The listing builds one solid part. Answer for the finished solid, in the listing's coordinates (mm). A direction names the side the tool comes from. Give positions to 0.01 mm unless a question says otherwise; leave off trailing zeros. Loops run counter-clockwise (first coordinate to the right, second up) from the corner with the lowest first, then second, coordinate; pieces in that order, holes last. Notation, with made-up numbers: M 47,39 L 84,39 A12 ccw 84,56 Z; hole C 83.5,62.5 d1. An arc over 180 degrees is marked long. One line per item, written item: value. Start each with the question number.
Q1. For faces 1 (the flat face through (77, 150, 3)), 2 (the flat face through (79, 170, 2)), determine the directions among +Z, -Z, +X, -X, +Y, -Y from which every point of the face is accessible in a straight line to the end or side of a thin tool.
Q2. A flat-ended cylindrical pin translates along its axis: pin 1 (4 mm diameter, centred on x = 160, y = 100, fed in from +Z). Find the tip coordinate at first contact, or state that the pin passes through.
Q3. A cutting plane is placed at B-B, the plane y = 22. Determine the outline of the cut face in (x, z).
Q4. Consider L1, parallel to X at y = 87.5, z = 2.6; L2, parallel to X at y = 132, z = 4.2; L3, parallel to Y at x = 40, z = 2.95. Determine where each line is inside the solid, lowest interval first.
Q5. The mould has two halves that part along X. Classify faces 3 (the flat face through (-15, 71, 2)), 4 (the flat face through (120, 69, 5)), 5 (the flat face through (45, 69, 3)): +X half, -X half, draft (parallel to the pull), parting line (faces both ways), or undercut.
Q6. A cutting plane is placed at C-C, the plane z = 2.95. State how many separate pieces and enclosed holes the cut face has, and give its area (3 significant figures).
Q7. A cutting plane is placed at A-A, the plane x = 56.5. Determine the outline of the cut face in (y, z), and give its area (3 significant figures).
from build123d import *

# Parameters (mm, degrees)
SKETCH_1_W          = 170
SKETCH_1_H          = 140
EXTRUDE_1_DEPTH     = 5
CUT_EXTRUDE_1_DEPTH = 5
SKETCH_4_R          = 1.6
CUT_EXTRUDE_2_DEPTH = 5
SKETCH_9_W          = 170
SKETCH_9_H          = 5
EXTRUDE_2_DEPTH     = 30
SKETCH_10_W         = 170
SKETCH_10_H         = 5
EXTRUDE_3_DEPTH     = 30
SKETCH_8_W          = 65
SKETCH_8_H          = 160
CUT_EXTRUDE_5_DEPTH = 30
SKETCH_6_R          = 1.75
CUT_EXTRUDE_6_DEPTH = 30
SKETCH_13_W         = 5
SKETCH_13_H         = 200
EXTRUDE_4_DEPTH     = 15
SKETCH_14_R         = 1.75
CUT_EXTRUDE_7_DEPTH = 15


with BuildPart() as part:
    # 草图1 → 凸台-拉伸1 (new body)
    with BuildSketch(Plane.XY):
        with Locations((85, 70)):
            Rectangle(SKETCH_1_W, SKETCH_1_H)
    extrude(amount=EXTRUDE_1_DEPTH)

    # 草图3 → 切除-拉伸1 (cut)
    with BuildSketch(Plane.XY.offset(5)):
        with BuildLine():
            ThreePointArc((10, 128.4), (11.13137085, 128.86862915), (11.6, 130))
            Line((11.6, 130), (10, 130))
            Line((10, 130), (10, 128.4))
        make_face()
        with BuildLine():
            Line((10, 130), (11.6, 130))
            ThreePointArc((11.6, 130), (8.86862915, 131.13137085), (10, 128.4))
            Line((10, 128.4), (10, 130))
        make_face()
        with BuildLine():
            ThreePointArc((10, 128.4), (11.13137085, 128.86862915), (11.6, 130))
            Line((11.6, 130), (10, 130))
            Line((10, 130), (10, 128.4))
        make_face()
        with BuildLine():
            Line((10, 130), (11.6, 130))
            ThreePointArc((11.6, 130), (8.86862915, 131.13137085), (10, 128.4))
            Line((10, 128.4), (10, 130))
        make_face()
        with BuildLine():
            ThreePointArc((11.6, 10), (11.13137085, 11.13137085), (10, 11.6))
            Line((10, 11.6), (10, 10))
            Line((10, 10), (11.6, 10))
        make_face()
        with BuildLine():
            Line((10, 10), (10, 11.6))
            ThreePointArc((10, 11.6), (8.86862915, 8.86862915), (11.6, 10))
            Line((11.6, 10), (10, 10))
        make_face()
        with BuildLine():
            ThreePointArc((11.6, 10), (11.13137085, 11.13137085), (10, 11.6))
            Line((10, 11.6), (10, 10))
            Line((10, 10), (11.6, 10))
        make_face()
        with BuildLine():
            Line((10, 10), (10, 11.6))
            ThreePointArc((10, 11.6), (8.86862915, 8.86862915), (11.6, 10))
            Line((11.6, 10), (10, 10))
        make_face()
        with BuildLine():
            ThreePointArc((161.6, 10), (161.13137085, 11.13137085), (160, 11.6))
            Line((160, 11.6), (160, 10))
            Line((160, 10), (158.4, 10))
            ThreePointArc((158.4, 10), (160, 8.4), (161.6, 10))
        make_face()
        with BuildLine():
            Line((160, 10), (160, 11.6))
            ThreePointArc((160, 11.6), (158.86862915, 11.13137085), (158.4, 10))
            Line((158.4, 10), (160, 10))
        make_face()
        with BuildLine():
            ThreePointArc((161.6, 10), (161.13137085, 11.13137085), (160, 11.6))
            Line((160, 11.6), (160, 10))
            Line((160, 10), (158.4, 10))
            ThreePointArc((158.4, 10), (160, 8.4), (161.6, 10))
        make_face()
        with BuildLine():
            Line((160, 10), (160, 11.6))
            ThreePointArc((160, 11.6), (158.86862915, 11.13137085), (158.4, 10))
            Line((158.4, 10), (160, 10))
        make_face()
        with BuildLine():
            ThreePointArc((161.6, 130), (160, 131.6), (158.4, 130))
            Line((158.4, 130), (160, 130))
            Line((160, 130), (160, 128.4))
            ThreePointArc((160, 128.4), (161.13137085, 128.86862915), (161.6, 130))
        make_face()
        with BuildLine():
            Line((160, 130), (158.4, 130))
            ThreePointArc((158.4, 130), (158.86862915, 128.86862915), (160, 128.4))
            Line((160, 128.4), (160, 130))
        make_face()
        with BuildLine():
            ThreePointArc((161.6, 130), (160, 131.6), (158.4, 130))
            Line((158.4, 130), (160, 130))
            Line((160, 130), (160, 128.4))
            ThreePointArc((160, 128.4), (161.13137085, 128.86862915), (161.6, 130))
        make_face()
        with BuildLine():
            Line((160, 130), (158.4, 130))
            ThreePointArc((158.4, 130), (158.86862915, 128.86862915), (160, 128.4))
            Line((160, 128.4), (160, 130))
        make_face()
    extrude(amount=-CUT_EXTRUDE_1_DEPTH, mode=Mode.SUBTRACT)

    # 草图4 → 切除-拉伸2 (cut)
    with BuildSketch(Plane.XY.offset(5)):
        with Locations((10, 130)):
            Circle(SKETCH_4_R)
        with Locations((40, 130)):
            Circle(SKETCH_4_R)
        with Locations((70, 130)):
            Circle(SKETCH_4_R)
        with Locations((100, 130)):
            Circle(SKETCH_4_R)
        with Locations((130, 130)):
            Circle(SKETCH_4_R)
        with Locations((10, 10)):
            Circle(SKETCH_4_R)
        with Locations((40, 10)):
            Circle(SKETCH_4_R)
        with Locations((70, 10)):
            Circle(SKETCH_4_R)
        with Locations((100, 10)):
            Circle(SKETCH_4_R)
        with Locations((130, 10)):
            Circle(SKETCH_4_R)
        with Locations((160, 130)):
            Circle(SKETCH_4_R)
        with Locations((10, 100)):
            Circle(SKETCH_4_R)
        with Locations((160, 100)):
            Circle(SKETCH_4_R)
        with Locations((10, 70)):
            Circle(SKETCH_4_R)
        with Locations((160, 70)):
            Circle(SKETCH_4_R)
        with Locations((10, 40)):
            Circle(SKETCH_4_R)
        with Locations((160, 40)):
            Circle(SKETCH_4_R)
    extrude(amount=-CUT_EXTRUDE_2_DEPTH, mode=Mode.SUBTRACT)

    # 草图9 → 凸台-拉伸2 (add)
    with BuildSketch(Plane.XZ):
        with Locations((85, 2.5)):
            Rectangle(SKETCH_9_W, SKETCH_9_H)
    extrude(amount=EXTRUDE_2_DEPTH)

    # 草图10 → 凸台-拉伸3 (add)
    with BuildSketch(Plane(origin=(0, 140, 0), x_dir=(1, 0, 0), z_dir=(0, 1, 0))):
        with Locations((85, -2.5)):
            Rectangle(SKETCH_10_W, SKETCH_10_H)
    extrude(amount=EXTRUDE_3_DEPTH)

    # 草图8 → 切除-拉伸5 (cut)
    with BuildSketch(Plane.XY.offset(5)):
        with Locations((77.5, 70)):
            Rectangle(SKETCH_8_W, SKETCH_8_H)
    extrude(amount=-CUT_EXTRUDE_5_DEPTH, mode=Mode.SUBTRACT)

    # 草图6 → 切除-拉伸6 (cut)
    with BuildSketch(Plane.XY.offset(5)):
        with Locations((123, 92)):
            Circle(SKETCH_6_R)
        with Locations((167, 92)):
            Circle(SKETCH_6_R)
        with Locations((123, 48)):
            Circle(SKETCH_6_R)
        with Locations((167, 48)):
            Circle(SKETCH_6_R)
    extrude(amount=-CUT_EXTRUDE_6_DEPTH, mode=Mode.SUBTRACT)

    # 草图13 → 凸台-拉伸4 (add)
    with BuildSketch(Plane.ZY):
        with Locations((2.5, 70)):
            Rectangle(SKETCH_13_W, SKETCH_13_H)
    extrude(amount=EXTRUDE_4_DEPTH)

    # 草图14 → 切除-拉伸7 (cut)
    with BuildSketch(Plane.XY.offset(5)):
        with BuildLine():
            ThreePointArc((-8.25, 152.5), (-11.237436867, 153.737436867), (-10, 150.75))
            Line((-10, 150.75), (-10, 152.5))
            Line((-10, 152.5), (-8.25, 152.5))
        make_face()
        with BuildLine():
            Line((-10, 152.5), (-10, 150.75))
            ThreePointArc((-10, 150.75), (-8.762563133, 151.262563133), (-8.25, 152.5))
            Line((-8.25, 152.5), (-10, 152.5))
        make_face()
        with BuildLine():
            ThreePointArc((-8.25, 152.5), (-11.237436867, 153.737436867), (-10, 150.75))
            Line((-10, 150.75), (-10, 152.5))
            Line((-10, 152.5), (-8.25, 152.5))
        make_face()
        with BuildLine():
            Line((-10, 152.5), (-10, 150.75))
            ThreePointArc((-10, 150.75), (-8.762563133, 151.262563133), (-8.25, 152.5))
            Line((-8.25, 152.5), (-10, 152.5))
        make_face()
        with BuildLine():
            Line((-10, 139.25), (-10, 137.5))
            Line((-10, 137.5), (-8.25, 137.5))
            ThreePointArc((-8.25, 137.5), (-8.762563133, 138.737436867), (-10, 139.25))
        make_face()
        with BuildLine():
            Line((-8.25, 137.5), (-10, 137.5))
            Line((-10, 137.5), (-10, 139.25))
            ThreePointArc((-10, 139.25), (-11.237436867, 136.262563133), (-8.25, 137.5))
        make_face()
        with BuildLine():
            Line((-10, 139.25), (-10, 137.5))
            Line((-10, 137.5), (-8.25, 137.5))
            ThreePointArc((-8.25, 137.5), (-8.762563133, 138.737436867), (-10, 139.25))
        make_face()
        with BuildLine():
            Line((-8.25, 137.5), (-10, 137.5))
            Line((-10, 137.5), (-10, 139.25))
            ThreePointArc((-10, 139.25), (-11.237436867, 136.262563133), (-8.25, 137.5))
        make_face()
        with BuildLine():
            ThreePointArc((18, 139.25), (16.762563133, 138.737436867), (16.25, 137.5))
            Line((16.25, 137.5), (18, 137.5))
            Line((18, 137.5), (18, 139.25))
        make_face()
        with BuildLine():
            Line((18, 137.5), (16.25, 137.5))
            ThreePointArc((16.25, 137.5), (18, 135.75), (19.75, 137.5))
            ThreePointArc((19.75, 137.5), (19.237436867, 138.737436867), (18, 139.25))
            Line((18, 139.25), (18, 137.5))
        make_face()
        with BuildLine():
            ThreePointArc((18, 139.25), (16.762563133, 138.737436867), (16.25, 137.5))
            Line((16.25, 137.5), (18, 137.5))
            Line((18, 137.5), (18, 139.25))
        make_face()
        with BuildLine():
            Line((18, 137.5), (16.25, 137.5))
            ThreePointArc((16.25, 137.5), (18, 135.75), (19.75, 137.5))
            ThreePointArc((19.75, 137.5), (19.237436867, 138.737436867), (18, 139.25))
            Line((18, 139.25), (18, 137.5))
        make_face()
        with BuildLine():
            ThreePointArc((16.25, 152.5), (16.762563133, 151.262563133), (18, 150.75))
            Line((18, 150.75), (18, 152.5))
            Line((18, 152.5), (16.25, 152.5))
        make_face()
        with BuildLine():
            Line((18, 152.5), (18, 150.75))
            ThreePointArc((18, 150.75), (19.237436867, 151.262563133), (19.75, 152.5))
            ThreePointArc((19.75, 152.5), (18, 154.25), (16.25, 152.5))
            Line((16.25, 152.5), (18, 152.5))
        make_face()
        with BuildLine():
            ThreePointArc((16.25, 152.5), (16.762563133, 151.262563133), (18, 150.75))
            Line((18, 150.75), (18, 152.5))
            Line((18, 152.5), (16.25, 152.5))
        make_face()
        with BuildLine():
            Line((18, 152.5), (18, 150.75))
            ThreePointArc((18, 150.75), (19.237436867, 151.262563133), (19.75, 152.5))
            ThreePointArc((19.75, 152.5), (18, 154.25), (16.25, 152.5))
            Line((16.25, 152.5), (18, 152.5))
        make_face()
        with Locations((-10, 102.5)):
            Circle(SKETCH_14_R)
        with Locations((18, 102.5)):
            Circle(SKETCH_14_R)
        with Locations((-10, 87.5)):
            Circle(SKETCH_14_R)
        with Locations((18, 87.5)):
            Circle(SKETCH_14_R)
        with Locations((-10, 52.5)):
            Circle(SKETCH_14_R)
        with Locations((18, 52.5)):
            Circle(SKETCH_14_R)
        with Locations((-10, 37.5)):
            Circle(SKETCH_14_R)
        with Locations((18, 37.5)):
            Circle(SKETCH_14_R)
        with Locations((-10, 2.5)):
            Circle(SKETCH_14_R)
        with Locations((18, 2.5)):
            Circle(SKETCH_14_R)
        with Locations((-10, -12.5)):
            Circle(SKETCH_14_R)
        with Locations((18, -12.5)):
            Circle(SKETCH_14_R)
    extrude(amount=-CUT_EXTRUDE_7_DEPTH, mode=Mode.SUBTRACT)


solid = part.part
Answer block:
1. face 1: +Z, -Z
1. face 2: +Z, -Z, +X, -X, +Y
2. pin 1: z = 5
3. outline: M -15,0 L 45,0 L 45,5 L -15,5 Z; M 110,0 L 170,0 L 170,5 L 110,5 Z
4. L1: -15 to -11.75, -8.25 to 16.25, 19.75 to 45, 110 to 170
4. L2: -15 to 45, 110 to 170
4. L3: -30 to 8.4, 11.6 to 128.4, 131.6 to 170
5. face 3: -X half
5. face 4: draft
5. face 5: undercut
6. separate pieces: 1
6. enclosed holes: 35
6. area: 26,300 mm^2
7. outline: M -30,0 L -10,0 L -10,5 L -30,5 Z; M 150,0 L 170,0 L 170,5 L 150,5 Z
7. area: 200 mm^2
